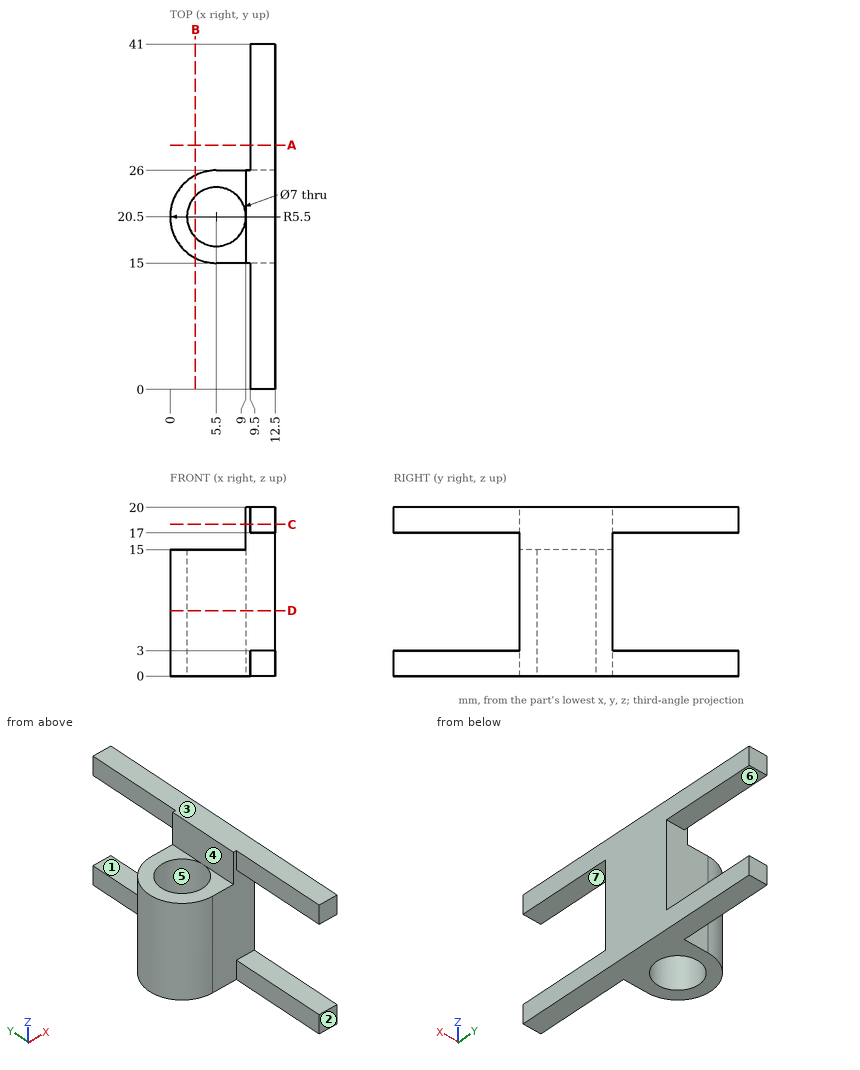
Geometry check sheet. Reference: drawing and pictorial views, mm from the part's lowest x, y, z. A direction names the side the tool comes from. Give positions to 0.01 mm unless a question says otherwise; leave off trailing zeros. Write each loop counter-clockwise with the first axis right and the second up, starting at its lowest first coordinate (ties: lowest second). Pieces come first, ordered by that corner, then holes. Notation, with made-up numbers: (21, 22.5) -> (60, 22.5) arc R12 cw to (60, 36.5) -> close; hole circle Ø4 at (25, 70). An arc over 180 degrees is marked (long way). One line per question, with ' | ' between items.
Item 1: Draft check along Z on the marked faces 1, 2 and 3. Enter one of: released by +Z, released by -Z, zero draft, split by the parting line, or undercut.
Determined:
face 1: undercut | face 2: zero draft | face 3: released by +Z
Item 2: Access from +Z, -Z, +X, -X, +Y, -Y to the whole of each face (thin tool, end or side, straight path). Record for the marked faces 4, 5, 6 and 7.
Determined:
face 4: +Z, -X, +Y, -Y | face 5: +Z, -Z | face 6: +X, -X, +Y | face 7: +X, -X, -Y
Item 3: Sectioned sample at D-D, the plane z = 7.75. Record the boundary of the cut face in (x, y), plus the area to 3 significant figures.
Determined:
outline: (5.5, 15) -> (12.5, 15) -> (12.5, 26) -> (5.5, 26) arc R5.5 ccw to start; hole circle Ø7 at (5.5, 20.5) | area: 86.0 mm^2
Item 4: Sectioned sample at C-C, the plane z = 18. Record the boundary of the cut face in (x, y), plus the area to 4 significant figures.
Determined:
outline: (9, 15) -> (9.5, 15) -> (9.5, 0) -> (12.5, 0) -> (12.5, 41) -> (9.5, 41) -> (9.5, 26) -> (9, 26) -> close | area: 128.5 mm^2
Item 5: Scan lines: line 1 along Y through (x, z) = (5.5, 12.25); line 2 along Y through (x, z) = (9.75, 9); line 3 along Y through (x, z) = (4, 12.5). Record each from-to range of solid material in increasing order.
Determined:
line 1: 15 to 17, 24 to 26 | line 2: 15 to 26 | line 3: 15.21 to 17.34, 23.66 to 25.79
Item 6: Depth check by flat-ended pin: pin 1 (2 mm diameter, centred on x = 10.5, z = 6.5, fed in from +Y); pin 2 (2.5 mm diameter, centred on y = 33.5, z = 19, fed in from -X); pin 3 (7.5 mm diameter, centred on x = 8.5, z = 8.5, fed in from -Y); pin 4 (3.5 mm diameter, centred on x = 11.5, y = 30.5, fed in from -Z). Enter the tip coordinate at first touch or a pass-through.
Determined:
pin 1: y = 26 | pin 2: x = 9.5 | pin 3: y = 15 | pin 4: z = 0
Item 7: Sectioned sample at A-A, the plane y = 29. Record the boundary of the cut face in (x, z).
Determined:
outline: (9.5, 0) -> (12.5, 0) -> (12.5, 3) -> (9.5, 3) -> close; (9.5, 17) -> (12.5, 17) -> (12.5, 20) -> (9.5, 20) -> close
Item 8: Sectioned sample at B-B, the plane x = 3. Record the boundary of the cut face in (y, z).
Determined:
outline: (15.6, 0) -> (18.05, 0) -> (18.05, 15) -> (15.6, 15) -> close; (22.95, 0) -> (25.4, 0) -> (25.4, 15) -> (22.95, 15) -> close
